CAD build for the part. Positions are in the model's coordinates, mm. A direction names the side the tool comes from. Round coordinates to 2 decimals unless told otherwise and drop trailing zeros. Order: outer loops, then holes, each group sorted by start corner. A loop starts at its lowest first (then second) coordinate and runs counter-clockwise, first axis right, second up. Notation, with made-up numbers: M -16.75,19 L -9.75,19 A27 cw -9.75,36 Z; hole C 23.25,78 d2. An arc over 180 degrees is marked long. Put each result on its own line as item: value.
```python
from build123d import *

# Parameters (mm, degrees)
SKETCH2_W           = 15.5
SKETCH2_H           = 14
BOSS_EXTRUDE1_DEPTH = 3
CIRPATTERN1_COUNT   = 3
CUT_EXTRUDE1_DEPTH  = 12
CUT_EXTRUDE2_START  = -9
CUT_EXTRUDE2_DEPTH  = 3
CUT_EXTRUDE3_REACH  = 60.279
SKETCH6_R           = 2.5
CIRPATTERN2_COUNT   = 3
FILLET1_R           = 1.5
CHAMFER1_SIZE       = 3
CHAMFER2_SIZE       = 1


with BuildPart() as part:
    # Sketch1 → Revolve1 (revolve)
    with BuildSketch(Plane.XY, mode=Mode.PRIVATE) as revolve1_sk:
        Polygon((0, 0), (35.5, 0), (35.5, 8), (15, 9.999206161), (15, 24), (0, 24), align=None)
    revolve(revolve1_sk.sketch.rotate(Axis((0, -5.176379432, 0), (0, 1, 0)), 90), axis=Axis((0, -5.176379432, 0), (0, 1, 0)))

    # Sketch2 → Boss-Extrude1 (add, symmetric)
    with BuildSketch(Plane.XY):
        with Locations((27.75, 14)):
            Rectangle(SKETCH2_W, SKETCH2_H)
    boss_extrude1 = extrude(amount=BOSS_EXTRUDE1_DEPTH, both=True)

    # CirPattern1: Boss-Extrude1 ×3 about axis
    cirpattern1_axis = Axis((0, 0, 0), (0, 1, 0))
    for i in range(1, CIRPATTERN1_COUNT):
        add(boss_extrude1.rotate(cirpattern1_axis, i * 360 / CIRPATTERN1_COUNT))

    # Sketch3 → Cut-Revolve1 (revolve, cut)
    with BuildSketch(Plane.XY, mode=Mode.PRIVATE) as cut_revolve1_sk:
        Polygon((0, 0), (22.5, 0), (22.5, 3), (7.5, 3), (7.5, 24), (0, 24), align=None)
    revolve(cut_revolve1_sk.sketch.rotate(Axis((0, -2.419018625, 0), (0, 1, 0)), 90), axis=Axis((0, -2.419018625, 0), (0, 1, 0)), mode=Mode.SUBTRACT)

    # Sketch4 → Cut-Extrude1 (cut)
    with BuildSketch(Plane.XZ.offset(-3)):
        with BuildLine():
            Line((-6.363961031, 8.485281374), (8.485281374, -6.363961031))
            ThreePointArc((8.485281374, -6.363961031), (8.485281374, -8.485281374), (6.363961031, -8.485281374))
            Line((6.363961031, -8.485281374), (-8.485281374, 6.363961031))
            ThreePointArc((-8.485281374, 6.363961031), (-8.485281374, 8.485281374), (-6.363961031, 8.485281374))
        make_face()
    extrude(amount=-CUT_EXTRUDE1_DEPTH, mode=Mode.SUBTRACT)

    # Sketch5 → Cut-Extrude2 (cut)
    with BuildSketch(Plane(origin=(0, 24, 0), x_dir=(1, 0, 0), z_dir=(0, 1, 0)).offset(CUT_EXTRUDE2_START)):
        with BuildLine():
            Line((9.492775288, 11.614095631), (4.135492251, 6.256812594))
            ThreePointArc((4.135492251, 6.256812594), (6.97813176, 2.7487592), (7.291643494, -1.755544118))
            Line((7.291643494, -1.755544118), (14.86337052, -2.019954652))
            ThreePointArc((14.86337052, -2.019954652), (13.95626352, 5.497518401), (9.492775288, 11.614095631))
        make_face()
        with BuildLine():
            Line((-4.135492251, -6.256812594), (-9.492775288, -11.614095631))
            ThreePointArc((-9.492775288, -11.614095631), (-13.95626352, -5.497518401), (-14.86337052, 2.019954652))
            Line((-14.86337052, 2.019954652), (-7.291643494, 1.755544118))
            ThreePointArc((-7.291643494, 1.755544118), (-6.97813176, -2.7487592), (-4.135492251, -6.256812594))
        make_face()
    extrude(amount=-CUT_EXTRUDE2_DEPTH, mode=Mode.SUBTRACT)

    # Sketch6 → Cut-Extrude3 (cut, up to next)
    with BuildSketch(Plane(origin=(-2.598076211, 0, -1.5), x_dir=(0.500000000000004, 0, -0.8660254037844364), z_dir=(0.8660254037844365, 0, 0.500000000000004)), mode=Mode.PRIVATE) as cut_extrude3_sk1:
        with Locations(Location((-30, 16, 0), (0, 0, 180))):
            Circle(SKETCH6_R)
    cut_extrude3_tool1 = extrude(cut_extrude3_sk1.sketch, amount=CUT_EXTRUDE3_REACH, mode=Mode.PRIVATE) & part.part
    cut_extrude3 = cut_extrude3_tool1.solids().sort_by_distance((-17.598076, 16, 24.480762))[0]
    add(cut_extrude3, mode=Mode.SUBTRACT)

    # CirPattern2: Cut-Extrude3 ×3 about axis
    cirpattern2_axis = Axis((0, -5.176379432, 0), (0, -1, 0))
    for i in range(1, CIRPATTERN2_COUNT):
        add(cut_extrude3.rotate(cirpattern2_axis, i * 360 / CIRPATTERN2_COUNT), mode=Mode.SUBTRACT)

    # Fillet1
    fillet1_edges = [part.edges().sort_by_distance(p)[0] for p in [
        (11.077507007, 15, 1.887749385),
        (11.077507007, 12, 1.887749385),
        (6.814133769, 15, -8.935454113),
        (7.928368159, 12, -10.049688503),
        (-6.814133769, 15, 8.935454113),
        (-7.928368159, 12, 10.049688503),
        (-11.077507007, 15, -1.887749385),
        (-11.077507007, 12, -1.887749385),
    ]]
    fillet(fillet1_edges, radius=FILLET1_R - 0.0001)  # a hair under: the kernel refuses the full size

    # Chamfer1
    chamfer1_edges = [part.edges().sort_by_distance(p)[0] for p in [
        (35.5, 21, 0),
        (20, 21, 0),
        (-17.75, 21, 30.743901834),
        (-10, 21, 17.320508076),
        (-17.75, 21, -30.743901834),
        (-10, 21, -17.320508076),
    ]]
    chamfer(chamfer1_edges, length=CHAMFER1_SIZE)

    # Chamfer2
    chamfer2_edges = [part.edges().sort_by_distance(p)[0] for p in [
        (0, 24, 15),
    ]]
    chamfer(chamfer2_edges, length=CHAMFER2_SIZE)


solid = part.part
```
Item 1: Band-saw the part on A-A on x = 0. Give the cut face in (y, z), and give its area (3 significant figures).
Answers below:
outline: M 0,-35.5 L 8,-35.5 L 10,-15 L 23,-15 L 24,-14 L 24,-7.5 L 3,-7.5 L 3,-22.5 L 0,-22.5 Z; M 0,22.5 L 3,22.5 L 3,7.5 L 24,7.5 L 24,14 L 23,15 L 10,15 L 8,35.5 L 0,35.5 Z
area: 638 mm²
Item 2: Band-saw the part on B-B on y = 16. Give the cut face in (x, z), and give its area (3 significant figures).
Answers below:
outline: M -20.35,-29.24 L -15.15,-32.24 L -13.65,-29.65 L -18.85,-26.65 Z; M -20.35,29.24 L -18.85,26.65 L -13.65,29.65 L -15.15,32.24 Z; M -16.35,-22.32 L -11.15,-25.32 L -7.4,-18.82 L -12.6,-15.82 Z; M -16.35,22.32 L -12.6,15.82 L -7.4,18.82 L -11.15,25.32 Z; C 0,0 d30; M 20,-3 L 27.5,-3 L 27.5,3 L 20,3 Z; M 32.5,-3 L 35.5,-3 L 35.5,3 L 32.5,3 Z; hole C 0,0 d15
area: 719 mm²
Item 3: Mould opens along Z. For faces 4 (the flat face through (-14, 21, -24)), 5 (the flat face through (-16.95, 19.52, -29.45)), 6 (the cylindrical face through (2.87, 13.65, -6.93)), 7 (the cylindrical face through (11.18, 12.45, 1.46)) say: pulls with the +Z half, pulls with the -Z half, needs draft (parallel to the pull), parting line crosses it, or undercut.
Answers below:
face 4: needs draft
face 5: pulls with the -Z half
face 6: undercut
face 7: undercut
Item 4: Band-saw the part on C-C on y = 5.5. Give the cut face in (x, z).
Answers below:
outline: C 0,0 d71; hole M -8.49,6.36 L -6.26,4.14 A7.5 ccw 4.14,-6.26 L 6.36,-8.49 A1.5 ccw 8.49,-6.36 L 6.26,-4.14 A7.5 ccw -4.14,6.26 L -6.36,8.49 A1.5 ccw Z
Item 5: Pin check, flat tips, straight feed: P1, Ø5, axis at x = 26.5, z = -0.5, coming from the +Y side; P2, Ø4, axis at x = 27.5, y = 17, coming from the +Z side; P3, Ø2, axis at y = 18.5, z = 13, coming from the -X side. Stop position of each tip, or through.
Answers below:
P1: y = 21
P2: z = 3
P3: x = -9
Item 6: Probe line 1 along X through (y, z) = (16, 0.25); line 2 along Z through (x, y) = (-12.5, 16.75); line 3 along X through (y, z) = (0.9, 0). List the from-to ranges inside material, lowest first. Write a range as [from, to].
Answers below:
line 1: [-15, -7.5], [7.5, 15], [20, 27.5], [32.5, 35.5]
line 2: [-24.67, -15.88], [-8.29, 8.29], [15.88, 24.67]
line 3: [-35.5, -22.5], [22.5, 35.5]
Item 7: Tool access for faces 1 (the flat face through (28, 14, 3)), 2 (the cylindrical face through (7.198, 14.572, -8.681)), 3 (the flat face through (10, 15, -4)): list every direction of +Z, -Z, +X, -X, +Y, -Y with a clear straight run to the whole face (end or side of a thin tool).
Answers below:
face 1: +Z, +X, +Y
face 2: +X
face 3: none
